from build123d import *

# Parameters (mm, degrees)
SKETCH1_R               = 8.89
BOSS_EXTRUDE1_DEPTH     = 7.9375
CHAMFER1_SIZE           = 0.381
CUT_EXTRUDE1_DEPTH      = 15.868359232
CUT_EXTRUDE1_DEPTH_BACK = 15.868359232
SKETCH3_R               = 1.905


with BuildPart() as part:
    # Sketch1 → Boss-Extrude1 (new, symmetric)
    with BuildSketch(Plane(origin=(0, 0, 0), x_dir=(1, 0, 0), z_dir=(0, 1, 0))):
        with Locations(Location((0, 0, 0), (0, 0, 270))):
            Circle(SKETCH1_R)
        Polygon((3.702835951, -6.4135), (7.405671903, 0), (3.702835951, 6.4135), (-3.702835951, 6.4135), (-7.405671903, 0), (-3.702835951, -6.4135), align=None, mode=Mode.SUBTRACT)
    extrude(amount=BOSS_EXTRUDE1_DEPTH, both=True)

    # Chamfer1
    chamfer1_edges = [part.edges().sort_by_distance(p)[0] for p in [
        (5.554253927, -7.9375, -3.20675),
        (0, -7.9375, -6.4135),
        (-5.554253927, -7.9375, -3.20675),
        (-5.554253927, -7.9375, 3.20675),
        (0, 7.9375, 6.4135),
        (5.554253927, 7.9375, 3.20675),
        (5.554253927, 7.9375, -3.20675),
        (0, 7.9375, -6.4135),
        (-5.554253927, 7.9375, -3.20675),
        (-5.554253927, 7.9375, 3.20675),
        (0, -7.9375, -8.89),
        (0, 7.9375, -8.89),
        (0, -7.9375, 6.4135),
        (5.554253927, -7.9375, 3.20675),
    ]]
    chamfer(chamfer1_edges, length=CHAMFER1_SIZE)

    # Sketch3 → Cut-Extrude1 (cut, two sides: drawn at the far end of the back side and taken through both)
    with BuildSketch(Plane.XY.offset(-CUT_EXTRUDE1_DEPTH_BACK)):
        with Locations((0, -2.9375)):
            Circle(SKETCH3_R)
        with Locations((0, 5.0625)):
            Circle(SKETCH3_R)
    extrude(amount=CUT_EXTRUDE1_DEPTH + CUT_EXTRUDE1_DEPTH_BACK, mode=Mode.SUBTRACT)


solid = part.part
Could you check a few things on this model? Use its own coordinates, in mm. A direction names the side the tool comes from. Give positions to 0.01 mm unless a question says otherwise; leave off trailing zeros. Loops run counter-clockwise (first coordinate to the right, second up) from the corner with the lowest first, then second, coordinate; pieces in that order, holes last. Notation, with made-up numbers: (22, 58.25) -> (42, 58.25) arc R19 ccw to (42, 76.25) -> close; hole circle Ø9 at (38.5, 8). An arc over 180 degrees is marked (long way). Answer as CSV lines item,"result". Start each with the question number.
(1) We'd pull the mould along Y, two halves only. Please class faces 1 (the flat face through (-5.58, 0.11, 3.16)), 2 (the cylindrical face through (-0.25, -1.05, -7.67)), 3 (the cylindrical face through (-1.903, -2.854, 7.634)), 4 (the flat face through (6, -7.938, 4)): released by +Y, released by -Y, zero draft, split by the parting line, or undercut.
(2) If we section it at C-C on y = -3.5: Write out the boundary of the cut face in (x, z), then the cut area to 3 significant figures.
(3) Which directions (+Z, -Z, +X, -X, +Y, -Y) give clear straight access to the entire face, cutting with the end or side of a thin tool? Please do faces 5 (the flat face through (5.689, 7.744, 3.348)), 6 (the flat face through (-5.694, -7.75, -3.351)), 7 (the flat face through (6, 7.938, 4)), 8 (the flat face through (5.5, 0.1, 3.3)).
(4) If we section it at A-A on x = 0: Count the separate pieces of the cut face and the enclosed holes in it, then the cut area to 3 significant figures.
(5) I need wall thicknesses on probe 1 along Y at (x, z) = (0, -8.1); probe 2 along Z at (x, y) = (-3, -5); probe 3 along X at (y, z) = (2.25, 6). Which ranges of each line are inside material? Lowest first, please.
(6) I'm going to push flat-ended pins straight in: pin 1 Ø3.5 at (x, y) = (1, -3) entering from +Z; pin 2 Ø2.5 at (x, y) = (0, -2.94) entering from +Z; pin 3 Ø8 at (x, y) = (6.5, 5) entering from +Z; pin 4 Ø1.5 at (x, y) = (6, 1.5) entering from -Z. Where does each tip first touch, or does it pass through?
(7) If we section it at B-B on y = 0.5: Write out the boundary of the cut face in (x, z), then the cut area to 3 significant figures.
Computed:
1,face 1,"zero draft"
1,face 2,"undercut"
1,face 3,"undercut"
1,face 4,"released by -Y"
2,outline,"(-7.41, 0) -> (-3.7, 6.41) -> (-1.82, 6.41) -> (-1.82, 8.7) arc R8.89 ccw to (-1.82, -8.7) -> (-1.82, -6.41) -> (-3.7, -6.41) -> close; (1.82, -8.7) arc R8.89 ccw to (1.82, 8.7) -> (1.82, 6.41) -> (3.7, 6.41) -> (7.41, 0) -> (3.7, -6.41) -> (1.82, -6.41) -> close"
2,area,"88.2 mm2"
3,face 5,"+Y"
3,face 6,"-Y"
3,face 7,"+Z, -Z, +X, -X, +Y"
3,face 8,"+Y, -Y"
4,separate pieces,"6"
4,enclosed holes,"0"
4,area,"40.3 mm2"
5,probe 1,"y = -7.94 to -4.84, -1.03 to 3.16, 6.97 to 7.94"
5,probe 2,"z = -8.37 to -6.41, 6.41 to 8.37"
5,probe 3,"x = -6.56 to -3.94, 3.94 to 6.56"
6,pin 1,"stops at z = 8.86"
6,pin 2,"passes through"
6,pin 3,"stops at z = 8.53"
6,pin 4,"stops at z = -7.17"
7,outline,"circle Ø17.78 at (0, 0); hole (-7.41, 0) -> (-3.7, -6.41) -> (3.7, -6.41) -> (7.41, 0) -> (3.7, 6.41) -> (-3.7, 6.41) -> close"
7,area,"106 mm2"
